The listing builds one solid part. Answer for the finished solid, in the listing's coordinates (mm). A direction names the side the tool comes from. Give positions to 0.01 mm unless a question says otherwise; leave off trailing zeros. Write each loop counter-clockwise with the first axis right and the second up, starting at its lowest first coordinate (ties: lowest second). Pieces come first, ordered by that corner, then holes. Notation, with made-up numbers: (48, 22.25) - (92, 22.25) arc R34 cw to (92, 59.25) - close; hole circle Ø2 at (-32.5, -34). An arc over 180 degrees is marked (long way). One line per item, written item: value. Start each with the question number.
from build123d import *

# Parameters (mm, degrees)
SKETCH1_W           = 65
SKETCH1_H           = 65
BOSS_EXTRUDE1_DEPTH = 70
SKETCH2_W           = 47
SKETCH2_H           = 47
CUT_EXTRUDE1_DEPTH  = 60
SKETCH3_W           = 32
SKETCH3_H           = 32
CUT_EXTRUDE2_DEPTH  = 60
SKETCH4_R           = 2.5
CUT_EXTRUDE3_DEPTH  = 15


with BuildPart() as part:
    # Sketch1 → Boss-Extrude1 (new body)
    with BuildSketch(Plane(origin=(0, 0, 0), x_dir=(1, 0, 0), z_dir=(0, 1, 0))):
        with Locations((32.5, 32.5)):
            Rectangle(SKETCH1_W, SKETCH1_H)
    extrude(amount=BOSS_EXTRUDE1_DEPTH)

    # Sketch2 → Cut-Extrude1 (cut)
    with BuildSketch(Plane(origin=(0, 70, 0), x_dir=(1, 0, 0), z_dir=(0, 1, 0))):
        with Locations((32.5, 32.5)):
            Rectangle(SKETCH2_W, SKETCH2_H)
    extrude(amount=-CUT_EXTRUDE1_DEPTH, mode=Mode.SUBTRACT)

    # Sketch3 → Cut-Extrude2 (cut)
    with BuildSketch(Plane.XZ):
        with Locations((32.5, -32.5)):
            Rectangle(SKETCH3_W, SKETCH3_H)
    extrude(amount=-CUT_EXTRUDE2_DEPTH, mode=Mode.SUBTRACT)

    # Sketch4 → Cut-Extrude3 (cut)
    with BuildSketch(Plane(origin=(0, 70, 0), x_dir=(1, 0, 0), z_dir=(0, 1, 0))):
        with Locations((4.5, 60.5)):
            Circle(SKETCH4_R)
        with Locations((60.5, 60.5)):
            Circle(SKETCH4_R)
        with Locations((60.5, 4.5)):
            Circle(SKETCH4_R)
        with Locations((4.5, 4.5)):
            Circle(SKETCH4_R)
    extrude(amount=-CUT_EXTRUDE3_DEPTH, mode=Mode.SUBTRACT)


solid = part.part
Item 1: Find section A-A on y = 21.5. Determine the outline of the cut face in (x, z).
Item 2: Find section C-C on x = 43. Determine the outline of the cut face in (y, z), plus the area to 3 significant figures.
Item 3: For faces 5 (the flat face through (32, 5, -48.5)), 6 (the flat face through (65, 35, -32)), 7 (the flat face through (32, 40, -56)), determine the directions among +Z, -Z, +X, -X, +Y, -Y from which every point of the face is accessible in a straight line to the end or side of a thin tool.
Item 4: The mould has two halves that part along Z. Classify faces 1 (the flat face through (32, 40, -9)), 2 (the flat face through (32, 35, -65)), 3 (the flat face through (0, 35, -32)), 4 (the flat face through (60, 55, -61)): +Z half, -Z half, draft (parallel to the pull), parting line (faces both ways), or undercut.
Item 5: Straight lines are drawn through the part: line 1 along X through (y, z) = (59, -4.5); line 2 along Z through (x, y) = (4.5, 60.75); line 3 along Z through (x, y) = (30, 46). For each, find the intervals that lie inside material, in ascending order.
Item 6: Each of these flat-tipped pins is pushed along its axis until it touches: pin 1 Ø2.5 at (x, z) = (4, -59.5) entering from +Y; pin 2 Ø23.5 at (x, z) = (22, -44) entering from +Y. Where does it stop, or does it pass through?
Item 7: Find section D-D on x = 6. Determine the outline of the cut face in (y, z).
Item 8: Find section B-B on z = -33. Determine the outline of the cut face in (x, y), plus the area to 3 significant figures.
Values:
1. outline: (0, -65) - (65, -65) - (65, 0) - (0, 0) - close; hole (9, -56) - (56, -56) - (56, -9) - (9, -9) - close
2. outline: (0, -65) - (70, -65) - (70, -56) - (10, -56) - (10, -48.5) - (0, -48.5) - close; (0, -16.5) - (10, -16.5) - (10, -9) - (70, -9) - (70, 0) - (0, 0) - close
2. area: 1,410 mm^2
3. face 5: +Y, -Y
3. face 6: +Z, -Z, +X, +Y, -Y
3. face 7: +Y
4. face 1: undercut
4. face 2: -Z half
4. face 3: draft
4. face 4: undercut
5. line 1: 0 to 2, 7 to 58, 63 to 65
5. line 2: -65 to -63, -58 to -7, -2 to 0
5. line 3: -65 to -56, -9 to 0
6. pin 1: y = 55
6. pin 2: y = 10
7. outline: (0, -65) - (70, -65) - (70, -62.5) - (55, -62.5) - (55, -58.5) - (70, -58.5) - (70, -6.5) - (55, -6.5) - (55, -2.5) - (70, -2.5) - (70, 0) - (0, 0) - close
8. outline: (0, 0) - (16.5, 0) - (16.5, 10) - (9, 10) - (9, 70) - (0, 70) - close; (48.5, 0) - (65, 0) - (65, 70) - (56, 70) - (56, 10) - (48.5, 10) - close
8. area: 1,410 mm^2
